from build123d import *

# Parameters (mm, degrees)
PAD_DEPTH = 8


with BuildPart() as part:
    # Sketch → Pad (new body)
    with BuildSketch(Plane.XY):
        with BuildLine():
            Line((4.25, -3.25), (4.25, -3.95))
            ThreePointArc((3.95, -4.25), (4.162132, -4.162132), (4.25, -3.95))
            Line((3.95, -4.25), (-3.95, -4.25))
            ThreePointArc((-4.25, -3.95), (-4.162132, -4.162132), (-3.95, -4.25))
            Line((-4.25, 3.95), (-4.25, -3.95))
            ThreePointArc((-3.95, 4.25), (-4.162132, 4.162132), (-4.25, 3.95))
            Line((-3.95, 4.25), (3.95, 4.25))
            ThreePointArc((4.25, 3.95), (4.162132, 4.162132), (3.95, 4.25))
            Line((4.25, 3.95), (4.25, 3.25))
            Line((4.25, 3.25), (6.25, 3.25))
            Line((6.25, 6.25), (6.25, 3.25))
            Line((6.25, 8.95), (6.25, 6.25))
            ThreePointArc((6.25, 8.95), (5.576346, 10.576346), (3.95, 11.25))
            Line((-1.45, 11.25), (3.95, 11.25))
            ThreePointArc((-1.45, 11.25), (-3.076346, 10.576346), (-3.75, 8.95))
            Line((-3.75, 8.95), (-3.75, 7.75))
            Line((-3.75, 7.75), (-1.75, 7.75))
            Line((-1.75, 8.95), (-1.75, 7.75))
            ThreePointArc((-1.45, 9.25), (-1.662132, 9.162132), (-1.75, 8.95))
            Line((3.95, 9.25), (-1.45, 9.25))
            ThreePointArc((4.25, 8.95), (4.162132, 9.162132), (3.95, 9.25))
            Line((4.25, 6.55), (4.25, 8.95))
            ThreePointArc((3.95, 6.25), (4.162132, 6.337868), (4.25, 6.55))
            Line((-3.95, 6.25), (3.95, 6.25))
            ThreePointArc((-3.95, 6.25), (-5.576346, 5.576346), (-6.25, 3.95))
            Line((-6.25, -3.95), (-6.25, 3.95))
            ThreePointArc((-6.25, -3.95), (-5.576346, -5.576346), (-3.95, -6.25))
            Line((3.95, -6.25), (-3.95, -6.25))
            ThreePointArc((3.95, -6.25), (5.576346, -5.576346), (6.25, -3.95))
            Line((6.25, -3.25), (6.25, -3.95))
            Line((4.25, -3.25), (6.25, -3.25))
        make_face()
    extrude(amount=PAD_DEPTH)


solid = part.part
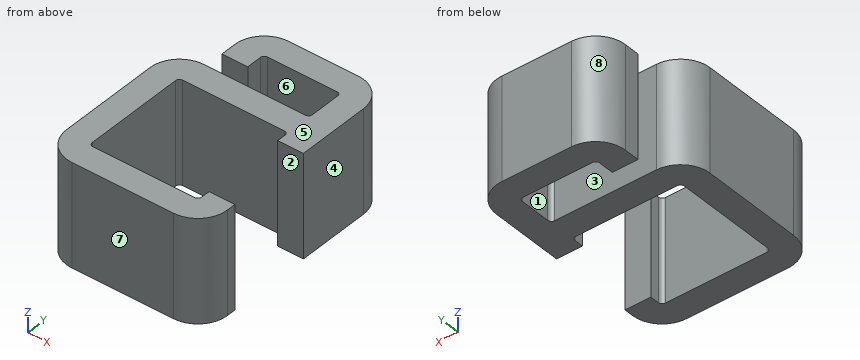
The listing builds one solid part. Answer for the finished solid, in the listing's coordinates (mm). Face numbers are marked on the shaded views. A direction names the side the tool comes from. Coordinates: 2 decimals unless noted, no trailing zeros. Write each loop counter-clockwise with the first axis right and the second up, starting at its lowest first coordinate (ties: lowest second). Pieces come first, ordered by that corner, then holes. Notation, with made-up numbers: M 66.5,41.25 L 82.5,41.25 A26 cw 82.5,72.25 Z; hole C 45,21.25 d2. An arc over 180 degrees is marked long. Put each result on its own line as item: value. Start each with the question number.
1. A cutting plane is placed at C-C on x = 5.5. Write down the section's boundary in (y, z), then the cut area to 3 significant figures.
2. For a pull along Y with two mould halves and no side action, classify the marked faces 5, 6, 7 and 8 as pulls with the +Y half, pulls with the -Y half, needs draft (parallel to the pull), parting line crosses it, or undercut.
3. Consider line 1 (Y direction, x = 3.75, z = 4.5); line 2 (X direction, y = 8.5, z = 0.5). Determine where each line is inside the solid, lowest interval first. Write a range as from..to.
4. Flat-ended cylindrical pins translate along their axes: P1, Ø2.5, axis at y = 8, z = 5, coming from the -X side; P2, Ø1.5, axis at x = -4, z = 1.5, coming from the +Y side; P3, Ø1.6, axis at x = 5, z = 4.5, coming from the -Y side. Find the tip coordinate at first contact, or state that the pin passes through.
5. A cutting plane is placed at D-D on x = -2.5. Write down the section's boundary in (y, z), then the cut area to 3 significant figures.
6. A cutting plane is placed at A-A on x = 0.25. Write down the section's boundary in (y, z).
7. Which of the six approach directions +Z, -Z, +X, -X, +Y, -Y give full straight-line access (tool end or side, diameter ignored) to the marked faces 1, 2, 3 and 4?
Resolved:
1. outline: M -5.65,0 L -3.25,0 L -3.25,8 L -5.65,8 Z; M 3.25,0 L 10.65,0 L 10.65,8 L 3.25,8 Z
1. area: 78.4 mm2
2. face 5: needs draft
2. face 6: undercut
2. face 7: pulls with the -Y half
2. face 8: pulls with the +Y half
3. line 1: y = -6.25..-4.25, 4.25..6.25, 9.25..11.25
3. line 2: x = -3.75..-1.75, 4.25..6.25
4. P1: stops at x = -3.75
4. P2: stops at y = 10.38
4. P3: stops at y = -6.24
5. outline: M -6.25,0 L -4.25,0 L -4.25,8 L -6.25,8 Z; M 4.25,0 L 6.25,0 L 6.25,8 L 4.25,8 Z; M 7.75,0 L 11,0 L 11,8 L 7.75,8 Z
5. area: 58.0 mm2
6. outline: M -6.25,0 L -4.25,0 L -4.25,8 L -6.25,8 Z; M 4.25,0 L 6.25,0 L 6.25,8 L 4.25,8 Z; M 9.25,0 L 11.25,0 L 11.25,8 L 9.25,8 Z
7. face 1: +Z, -Z
7. face 2: +Z, -Z, +X
7. face 3: +Z, -Z, -X
7. face 4: +Z, -Z, +X, +Y, -Y
